from build123d import *

# Parameters (mm, degrees)
BOSS_EXTRUDE1_DEPTH = 25.4
SKETCH2_R           = 9.801448676
SKETCH2_R_2         = 7.071368029
BOSS_EXTRUDE2_DEPTH = 19
BOSS_EXTRUDE3_DEPTH = 3.175
SKETCH4_R           = 3.175
CUT_EXTRUDE1_DEPTH  = 3.175


with BuildPart() as part:
    # Sketch1 → Boss-Extrude1 (new body)
    with BuildSketch(Plane.XY):
        Polygon((-92.495819173, -3.422180745), (-20.941461675, -3.422180745), (-1.20885062, 35.305249012), (-7.464460479, 16.03438497), (-18.995819173, -6.597180745), (-92.495819173, -6.597180745), align=None)
    extrude(amount=BOSS_EXTRUDE1_DEPTH)

    # Sketch2 → Boss-Extrude2 (add)
    with BuildSketch(Plane(origin=(0, -3.422180745, 0), x_dir=(1, 0, 0), z_dir=(0, 1, 0))):
        with Locations((-92.495819173, -12.7)):
            Circle(SKETCH2_R)
        with Locations((-92.495819173, -12.7)):
            Circle(SKETCH2_R_2, mode=Mode.SUBTRACT)
    extrude(amount=-BOSS_EXTRUDE2_DEPTH)

    # Sketch3 → Boss-Extrude3 (add)
    with BuildSketch(Plane(origin=(0, -3.422180745, 0), x_dir=(1, 0, 0), z_dir=(0, 1, 0))):
        with BuildLine():
            Line((-98.728601618, -16.040159995), (-98.728601618, -9.359840005))
            ThreePointArc((-98.728601618, -9.359840005), (-99.567187202, -12.7), (-98.728601618, -16.040159995))
        make_face()
        with BuildLine():
            Line((-98.728601618, -9.359840005), (-98.728601618, -5.135555597))
            Line((-98.728601618, -5.135555597), (-102.297267848, -12.7))
            Line((-102.297267848, -12.7), (-98.728601618, -20.264444403))
            Line((-98.728601618, -20.264444403), (-98.728601618, -16.040159995))
            ThreePointArc((-98.728601618, -16.040159995), (-99.567187202, -12.7), (-98.728601618, -9.359840005))
        make_face()
        with BuildLine():
            ThreePointArc((-92.495819173, -2.898551324), (-95.806852438, -3.474738223), (-98.728601618, -5.135555597))
            Line((-98.728601618, -5.135555597), (-98.728601618, -9.359840005))
            ThreePointArc((-98.728601618, -9.359840005), (-96.12794976, -6.632721104), (-92.495819173, -5.628631971))
            Line((-92.495819173, -5.628631971), (-92.495819173, -2.898551324))
        make_face()
        with BuildLine():
            ThreePointArc((-92.495819173, -19.771368029), (-96.12794976, -18.767278896), (-98.728601618, -16.040159995))
            Line((-98.728601618, -16.040159995), (-98.728601618, -20.264444403))
            ThreePointArc((-98.728601618, -20.264444403), (-95.806852438, -21.925261777), (-92.495819173, -22.501448676))
            Line((-92.495819173, -22.501448676), (-92.495819173, -19.771368029))
        make_face()
        with BuildLine():
            ThreePointArc((-92.495819173, -22.501448676), (-95.806852438, -21.925261777), (-98.728601618, -20.264444403))
            Line((-98.728601618, -20.264444403), (-92.495819173, -25.4))
            Line((-92.495819173, -25.4), (-92.495819173, -22.501448676))
        make_face()
        with BuildLine():
            ThreePointArc((-92.495819173, -5.628631971), (-96.12794976, -6.632721104), (-98.728601618, -9.359840005))
            Line((-98.728601618, -9.359840005), (-98.728601618, -16.040159995))
            ThreePointArc((-98.728601618, -16.040159995), (-96.12794976, -18.767278896), (-92.495819173, -19.771368029))
            Line((-92.495819173, -19.771368029), (-92.495819173, -5.628631971))
        make_face()
        with BuildLine():
            Line((-92.495819173, -2.898551324), (-92.495819173, 0))
            Line((-92.495819173, 0), (-98.728601618, -5.135555597))
            ThreePointArc((-98.728601618, -5.135555597), (-95.806852438, -3.474738223), (-92.495819173, -2.898551324))
        make_face()
    extrude(amount=-BOSS_EXTRUDE3_DEPTH)

    # Sketch4 → Cut-Extrude1 (cut)
    with BuildSketch(Plane(origin=(-15.240970814, 7.765662505, 0), x_dir=(0, 0, 1), z_dir=(-0.891006524, 0.4539905, 0))):
        with Locations((12.7, 18.20840051)):
            Circle(SKETCH4_R)
    extrude(amount=-CUT_EXTRUDE1_DEPTH, mode=Mode.SUBTRACT)


solid = part.part
Build history of the part. All positions in model axes, mm. A direction names the side the tool comes from. Give positions to 0.01 mm unless a question says otherwise; leave off trailing zeros. Order: outer loops, then holes, each group sorted by start corner. A loop starts at its lowest first (then second) coordinate and runs counter-clockwise, first axis right, second up. Notation, with made-up numbers: M 71.5,-25 L 76.5,-25 A14 ccw 76.5,-10 Z; hole C 57.25,15 d8. An arc over 180 degrees is marked long. Use one line per item in the form item = value.
1) Tool access for faces 1 (the face through (-13.15, 4.88, 12.52)), 2 (the face through (-62, -3.422, 13)), 3 (the face through (-92, -6.597, 13)): list every direction of +Z, -Z, +X, -X, +Y, -Y with a clear straight run to the whole face (end or side of a thin tool).
Calculated:
face_1 = +Z, -Z, +X, -Y
face_2 = +Z, -Z, -X, +Y
face_3 = -Y
2) Drop flat-ended pins along their axis: pin 1 (8 mm diameter, centred on y = 1, z = 8, fed in from +X); pin 2 (2 mm diameter, centred on x = -65.5, z = 8, fed in from -Y); pin 3 (2 mm diameter, centred on x = -77.5, z = 20, fed in from +Y). Give the stop position or say it passes through.
Calculated:
pin_1 = -13.09
pin_2 = -6.6
pin_3 = -3.42
3) Two-plate mould, pull along Z, no slides. Class faces 4 (the face through (-95.569, -4.987, 2.532)), 5 (the face through (-51, -6.597, 13)), 6 (the face through (-102.288, -14.9, 12.269)), 7 (the face through (-85.964, -14.399, 15.408)): released by +Z, released by -Z, zero draft, split by the parting line, or undercut.
Calculated:
face_4 = released by -Z
face_5 = zero draft
face_6 = split by the parting line
face_7 = undercut
4) Saw through at D-D (y = 2.5). Give the cut face in (x, z).
Calculated:
outline = M -17.92,0 L -14.36,0 L -14.36,25.4 L -17.92,25.4 Z
5) Saw through at A-A (z = 12.7). Give the cut face in (x, y), plus the area to 3 significant figures.
Calculated:
outline = M -102.3,-22.42 L -99.57,-22.42 L -99.57,-6.6 L -85.42,-6.6 L -85.42,-22.42 L -82.69,-22.42 L -82.69,-6.6 L -19,-6.6 L -7.46,16.03 L -6.17,20.02 L -8.42,21.16 L -20.94,-3.42 L -102.3,-3.42 Z; M -5.53,26.82 L -4.19,26.13 L -1.21,35.31 Z
area = 444 mm2
6) Saw through at B-B (x = -91.5). Give the cut face in (y, z), plus the area to 3 significant figures.
Calculated:
outline = M -22.42,2.95 L -6.6,2.95 L -6.6,0 L -3.42,0 L -3.42,25.4 L -6.6,25.4 L -6.6,22.45 L -22.42,22.45 L -22.42,19.7 L -6.6,19.7 L -6.6,5.7 L -22.42,5.7 Z
area = 168 mm2
7) Probe probe 1 along X at (y, z) = (-13.75, 12.7); probe 2 along Y at (x, z) = (-62.5, 22.5); probe 3 along Y at (x, z) = (-98, 6.5). List the from-to ranges inside material, lowest first.
Calculated:
probe_1 = -102.3 to -99.57, -85.42 to -82.69
probe_2 = -6.6 to -3.42
probe_3 = -22.42 to -3.42
8) Saw through at C-C (z = 18.25). Give the cut face in (x, y).
Calculated:
outline = M -100.57,-22.42 L -96.88,-22.42 L -96.88,-6.6 L -88.11,-6.6 L -88.11,-22.42 L -84.42,-22.42 L -84.42,-6.6 L -19,-6.6 L -7.46,16.03 L -1.21,35.31 L -20.94,-3.42 L -100.57,-3.42 Z
